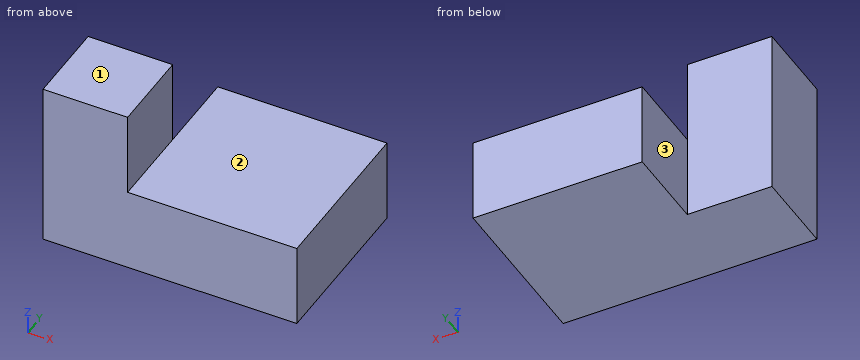
```python
from build123d import *

# Parameters (mm, degrees)
F1_DEPTH = 19.05
F2_W     = 38.1
F2_H     = 19.05
F3_DEPTH = 19.05


with BuildPart() as f1:
    # F0 (on Front) → F1 (new body)
    with BuildSketch(Plane.XZ):
        Polygon((-25.4, 19.05), (-25.4, -19.05), (31.75, -19.05), (31.75, 0), (-6.35, 0), (-6.35, 19.05), align=None)
    extrude(amount=F1_DEPTH)

    # F2 (on face) → F3 (join)
    with BuildSketch(Plane(origin=(0, 0, 0), x_dir=(-1, 0, 0), z_dir=(0, 1, 0))):
        with Locations((-12.7, -9.525)):
            Rectangle(F2_W, F2_H)
    extrude(amount=F3_DEPTH)


solid = f1.part
```
Could you check a few things on this model? Use its own coordinates, in mm. Face numbers are marked on the shaded views. A direction names the side the tool comes from. Round coordinates to 2 decimals unless told otherwise and drop trailing zeros. Loops run counter-clockwise (first coordinate to the right, second up) from the corner with the lowest first, then second, coordinate; pieces in that order, holes last.
Q1. I want a section at C-C (x = 12.5). Write out the boundary of the cut face in (y, z).
Q2. For P1, Ø15, axis at y = 12, z = -11.5, coming from the -X side; P2, Ø11.5, axis at x = 15.5, y = 9.5, coming from the +Z side; P3, Ø15, axis at y = -5.5, z = 11, coming from the +X side, each with a flat end and sliding along its axis, tell me the tip position at first contact or that it passes through.
Q3. I want a section at D-D (z = 7). Write out the boundary of the cut face in (x, y), and give its area (3 significant figures).
Q4. Please list where these lines run through material, in increasing order: L1, parallel to X at y = 7, z = -13.5; L2, parallel to Z at x = -2.5, y = -16.5; L3, parallel to X at y = -4, z = 14.5.
Q5. On a 3-axis mill with a long thin cutter (end or side, diameter ignored), from which of +Z, -Z, +X, -X, +Y, -Y can I reach the whole of each face in a straight line? I mean the marked faces 1, 2 and 3. Say none if no direction works.
Q6. I want a section at B-B (z = -12). Write out the boundary of the cut face in (x, y), and give its area (3 significant figures).
Q7. I want a section at A-A (y = -14.5). Write out the boundary of the cut face in (x, z), and give its area (3 significant figures).
Answer below:
1. outline: (-19.05, -19.05) - (19.05, -19.05) - (19.05, 0) - (-19.05, 0) - close
2. P1: stops at x = -6.35
2. P2: stops at z = 0
2. P3: stops at x = -6.35
3. outline: (-25.4, -19.05) - (-6.35, -19.05) - (-6.35, 0) - (-25.4, 0) - close
3. area: 363 mm2
4. L1: x = -6.35 to 31.75
4. L2: z = -19.05 to 0
4. L3: x = -25.4 to -6.35
5. face 1: +Z, +X, -X, +Y, -Y
5. face 2: +Z, +X, +Y, -Y
5. face 3: +Z, -Z, -X, +Y
6. outline: (-25.4, -19.05) - (31.75, -19.05) - (31.75, 19.05) - (-6.35, 19.05) - (-6.35, 0) - (-25.4, 0) - close
6. area: 1,810 mm2
7. outline: (-25.4, -19.05) - (31.75, -19.05) - (31.75, 0) - (-6.35, 0) - (-6.35, 19.05) - (-25.4, 19.05) - close
7. area: 1,450 mm2
